Autodesk Inventor part; units mm, degrees
ref_plane "YZ Plane" through (0, 0, 0) normal (1, 0, 0) x (0, 1, 0)
ref_plane "XZ Plane" through (0, 0, 0) normal (0, 1, 0) x (-1, 0, 0)
ref_plane "XY Plane" through (0, 0, 0) normal (0, 0, 1) x (1, 0, 0)
sketch "Skizze1" plane through (0, 0, 0) normal (0, 0, 1) x (1, 0, 0)
  line L0 (0, 0) -> (500, 0)
  line L1 (500, 0) -> (500, 144)
  line L2 (500, 144) -> (0, 144)
  line L3 (0, 144) -> (0, 0)
  line L4 (0, 25) -> (500, 25) construction
  line L5 (0, 50) -> (500, 50) construction
  line L6 (250, 0) -> (250, 144) construction
  line L7 (125, 0) -> (125, 144) construction
  line L8 (375, 144) -> (375, 0) construction
  circle A0 centre (125, 50) radius 2.5
  circle A1 centre (375, 50) radius 2.5
  circle A2 centre (375, 25) radius 3.5
  circle A3 centre (125, 25) radius 3.5
  line L9 (492, 144) -> (492, 0) construction
  line L10 (500, 112) -> (0, 112) construction
  line L11 (500, 32) -> (0, 32) construction
  circle A4 centre (492, 112) radius 1.5
  circle A5 centre (492, 32) radius 1.5
  line L12 (8, 144) -> (8, 0) construction
  circle A6 centre (8, 112) radius 1.5
  circle A7 centre (8, 72) radius 1.5
  circle A8 centre (8, 32) radius 1.5
  circle A9 centre (492, 72) radius 1.5
  point P0 (-875, 50)
  point P1 (-875, 25)
  point P2 (500, 72)
  dimension "d0" = 500
  dimension "d1" = 144
  dimension "d2" = 25
  dimension "d3" = 50
  dimension "d4" = 125
  dimension "d5" = 125
  dimension "d9" = 5
  dimension "d10" = 5
  dimension "d13" = 7
  dimension "d14" = 7
  dimension "d20" = 8
  dimension "d21" = 40
  dimension "d22" = 40
  dimension "d23" = 3
  dimension "d24" = 3
  dimension "d25" = 8
  dimension "d26" = 3
  dimension "d27" = 3
  dimension "d28" = 3
  dimension "d29" = 3
extrude "Extrusion1" add sketch "Skizze1" along normal blind 16
hole "Bohrung1" at (375, 25, 0) at (125, 25, 0) at (-875, 25, 0) direction (0, 0, 1) diameter 10 depth 12 tip angle 118
hole "Bohrung4" at (375, 50, 0) at (125, 50, 0) direction (0, 0, 1) diameter 7 depth 12 tip angle 118
sketch "Skizze2" plane through (0, 0, 16) normal (0, 0, 1) x (1, 0, 0)
  circle A0 centre (250, 72) radius 1.5
  circle A1 centre (492, 112) radius 1.5
  circle A2 centre (492, 72) radius 1.5
  circle A3 centre (492, 32) radius 1.5
  circle A4 centre (8, 72) radius 1.5
  circle A5 centre (8, 112) radius 1.5
  circle A6 centre (8, 32) radius 1.5
  circle A7 centre (250, 32) radius 1.5
  circle A8 centre (250, 112) radius 1.5
  point P0 (0, 0)
hole "Bohrung7" at (492, 112, 16) at (492, 72, 16) at (492, 32, 16) at (8, 72, 16) at (8, 32, 16) at (8, 112, 16) direction (0, 0, -1) diameter 3 depth 8 countersink diameter 8 countersink angle 90
sketch "Skizze3" plane through (0, 144, 0) normal (0, 1, 0) x (1, 0, 0)
  line L0 (500, -16) -> (0, -16) construction
  line L1 (0, -16) -> (0, 0) construction
  line L2 (0, 0) -> (500, 0) construction
  line L3 (500, 0) -> (500, -16) construction
  line L4 (500, -8) -> (0, -8) construction
  line L5 (0, 0) -> (0, -16) construction
  line L6 (0, -16) -> (500, -16) construction
  line L7 (460, -16) -> (460, 0) construction
  line L8 (0, 0) -> (500, 0) construction
  line L9 (40, -16) -> (40, 0) construction
  line L10 (250, -16) -> (250, 0) construction
  point P0 (460, -8)
  point P1 (250, -8)
  point P2 (40, -8)
  dimension "d120" = 40
  dimension "d121" = 40
hole "Bohrung12" at (460, 144, 8) at (250, 144, 8) at (40, 144, 8) direction (0, -1, 0) diameter 3 depth 30 tip angle 118
properties part number "licht_2m"
Verification items for the finished model (mm, model axes). A direction names the side the tool comes from. Round coordinates to 2 decimals unless told otherwise and drop trailing zeros. Use a Markdown table: item, result. Add a question column.
1. Thickness scan on probe 1 along Y at (x, z) = (125, 14); probe 2 along X at (y, z) = (25, 9.25); probe 3 along Y at (x, z) = (492, 5). Record the ranges inside material, lowest first. Write a range as [from, to].
2. Access from +Z, -Z, +X, -X, +Y, -Y to the whole of each face (thin tool, end or side, straight path). Record for faces 4 (the face through (125, 20, 6)), 5 (the face through (247, 0, 8)).
3. Gauge pin test, flat ends, axial feed: pin 1 (4 mm diameter, centred on x = 125, y = 50, fed in from -Z); pin 2 (5.5 mm diameter, centred on x = 125, y = 50, fed in from -Z); pin 3 (2.5 mm diameter, centred on x = 40, z = 8, fed in from +Y). Record the tip position at first contact, or that the pin passes through.
4. Release check for a two-part mould opening along Y. For faces 1 (the face through (7.366, 110.47, 13.656)), 2 (the face through (253, 144, 8)), 3 (the face through (0, 73, 8)) record: released by +Y, released by -Y, zero draft, split by the parting line, or undercut.
Checks:
| question | item | result |
|---|---|---|
| 1 | probe 1 | y = [0, 21.5], [28.5, 47.5], [52.5, 144] |
| 1 | probe 2 | x = [0, 120], [130, 370], [380, 500] |
| 1 | probe 3 | y = [0, 30.5], [33.5, 70.5], [73.5, 110.5], [113.5, 144] |
| 2 | face 4 | -Z |
| 2 | face 5 | +Z, -Z, +X, -X, -Y |
| 3 | pin 1 | passes through |
| 3 | pin 2 | stops at z = 12.45 |
| 3 | pin 3 | stops at y = 113.85 |
| 4 | face 1 | undercut |
| 4 | face 2 | released by +Y |
| 4 | face 3 | zero draft |
